Autodesk Inventor part; units mm, degrees
ref_plane "YZ Plane" through (0, 0, 0) normal (1, 0, 0) x (0, 1, 0)
ref_plane "XZ Plane" through (0, 0, 0) normal (0, 1, 0) x (-1, 0, 0)
sketch "Skizze1" plane through (0, 0, 0) normal (0, 0, 1) x (1, 0, 0)
  line L0 (0, 0) -> (0, 5)
  line L1 (0, 5) -> (0.8, 5)
  line L2 (0.8, 5) -> (0.8, 4.8)
  line L3 (0.8, 4.8) -> (1.9, 4.8)
  line L4 (1.9, 4.8) -> (1.9, 5)
  line L5 (1.9, 5) -> (34.9, 5)
  line L6 (34.9, 5) -> (34.9, 7.25)
  line L7 (34.9, 7.25) -> (40.9, 7.25)
  line L8 (40.9, 7.25) -> (40.9, 5)
  line L9 (40.9, 5) -> (73.9, 5)
  line L10 (73.9, 5) -> (73.9, 4.8)
  line L11 (73.9, 4.8) -> (75, 4.8)
  line L12 (75, 4.8) -> (75, 5)
  line L13 (75, 5) -> (75.8, 5)
  line L14 (75.8, 5) -> (75.8, 3)
  line L15 (75.8, 3) -> (83.8, 3)
  line L16 (83.8, 3) -> (83.8, 0)
  line L17 (83.8, 0) -> (0, 0)
  line L18 (25.9, 5) -> (25.9, 0) construction
  line L19 (49.9, 5) -> (49.9, 0) construction
  line L20 (15.9, 5) -> (15.9, 0) construction
  line L21 (59.9, 5) -> (59.9, 0) construction
  dimension "d0" = 10
  dimension "d1" = 6
  dimension "d2" = 14.5
  dimension "d3" = 1.1
  dimension "d4" = 9.6
  dimension "d5" = 0.8
  dimension "d6" = 0.8
  dimension "d7" = 9
  dimension "d8" = 9
  dimension "d9" = 6
  dimension "d10" = 24
  dimension "d11" = 24
  dimension "d12" = 8
  dimension "ParrallelMecha_DrivenLink_OuterWidth" = 72
  dimension "d22" = 10
  dimension "d23" = 10
  dimension "Querstrebe_Length" = 44
revolve "Umdrehung1" add sketch "Skizze1" angle 360 about axis through (83.8, 0, 0) along (-1, 0, 0)
chamfer "Fase1" distance 0.2 angle 45 5 edges at (34.9, -7.25, 0) (40.9, -7.25, 0) (75.8, -5, 0) (83.8, -3, 0) (0, -5, 0)
ref_plane "Wellennut_Spiegelebene" through (37.9, 0, 0) normal (-1, 0, 0) x (0, 0, 1)
ref_plane "Arbeitsebene2" through (18.4, 0, 5) normal (0, 0, 1) x (1, 0, 0)
sketch "Skizze3" plane through (18.4, 0, 5) normal (0, 0, 1) x (1, 0, 0)
  line L0 (7.5, 5) -> (7.5, 0) construction
  line L1 (-35.16, 0) -> (82.16, 0) construction
  line L2 (2, 0) -> (-11, 0) construction
  line L3 (2, 1.5) -> (-11, 1.5)
  line L4 (-11, -1.5) -> (2, -1.5)
  arc A0 (2, -1.5) -> (2, 1.5) centre (2, 0) ccw
  arc A1 (-11, 1.5) -> (-11, -1.5) centre (-11, 0) ccw
  line L5 (-16.5, 0) -> (7.5, 0) construction
  line L6 (-16.5, -5) -> (-16.5, 5) construction
  point P0 (-18.4, 0)
  point P1 (-4.5, 0)
  point P2 (-4.5, 0)
  dimension "d17" = 3
  dimension "d18" = 16
extrude "Wellennut" cut sketch "Skizze3" against normal blind 1.8
mirror "Spiegeln1" about plane through (37.9, 0, 0) normal (-1, 0, 0) of "Wellennut"
equation "\"d10\" = ParallelLink_Lever_Thickness_1 + ParallelLink_BearingStep_Height_1"
equation "\"d11\" = d10"
equation "\"d22\" = ParallelLink_BearingStep_Height_1"
equation "\"d23\" = d22"
properties part number "ParallelSystem_ProximalPart_Shaft_Driven" material "Edelstahl"
Work out the finished part from the listing and answer in its coordinate system (mm). A direction names the side the tool comes from. Give positions to 0.01 mm unless a question says otherwise; leave off trailing zeros. Loops run counter-clockwise (first coordinate to the right, second up) from the corner with the lowest first, then second, coordinate; pieces in that order, holes last. Notation, with made-up numbers: (48.25, -13) -> (56.25, -13) arc R13 ccw to (56.25, 10) -> close; hole circle Ø6 at (20.25, 53.5). An arc over 180 degrees is marked (long way). Put each result on its own line as item: value. Start each with the question number.
Item 1: Which of the six approach directions +Z, -Z, +X, -X, +Y, -Y give full straight-line access (tool end or side, diameter ignored) to faces 4 (the face through (80, -3, 0)), 5 (the face through (1.36, 2.58, 4.05)), 6 (the face through (14, -1.5, 4))?
Item 2: Find the intervals of material crossed by L1, parallel to Z at x = 65, y = -0.25; L2, parallel to X at y = -3.5, z = 0.5; L3, parallel to X at y = 5.25, z = 0.75, in increasing order. Write a range as [from, to].
Item 3: The part is cut by section A-A (x = 65.5). Give the vertices of the cut face in (y, z).
Item 4: Each of these flat-tipped pins is pushed along its axis until it touches: P1, Ø1.5, axis at x = 60.5, y = 0, coming from the +Z side; P2, Ø2.5, axis at x = 11.5, y = 0.5, coming from the +Z side; P3, Ø1.7, axis at x = 12.5, z = 4, coming from the +Y side. Where does it stop, or does it pass through?
Item 5: The mould has two halves that part along X. Classify faces 1 (the face through (14, 0, 3.2)), 2 (the face through (0.5, -1.08, -4.88)), 3 (the face through (75.8, 1, 3)): released by +X, released by -X, zero draft, split by the parting line, or undercut.
Item 6: The part is cut by section B-B (x = 48). Give the vertices of the cut face in (y, z), then the cut area to 3 significant figures.
Answers below:
1. face 4: +X
1. face 5: none
1. face 6: +Z
2. L1: [-4.99, 3.2]
2. L2: [0, 75.8]
2. L3: [34.9, 40.9]
3. outline: (-1.5, 3.2) -> (-1.5, 4.77) arc R5 ccw (long way) to (1.5, 4.77) -> (1.5, 3.2) -> close
4. P1: z = 3.2
4. P2: z = 4.77
4. P3: y = 3.88
5. face 1: undercut
5. face 2: zero draft
5. face 3: released by +X
6. outline: circle Ø10 at (0, 0)
6. area: 78.5 mm2
